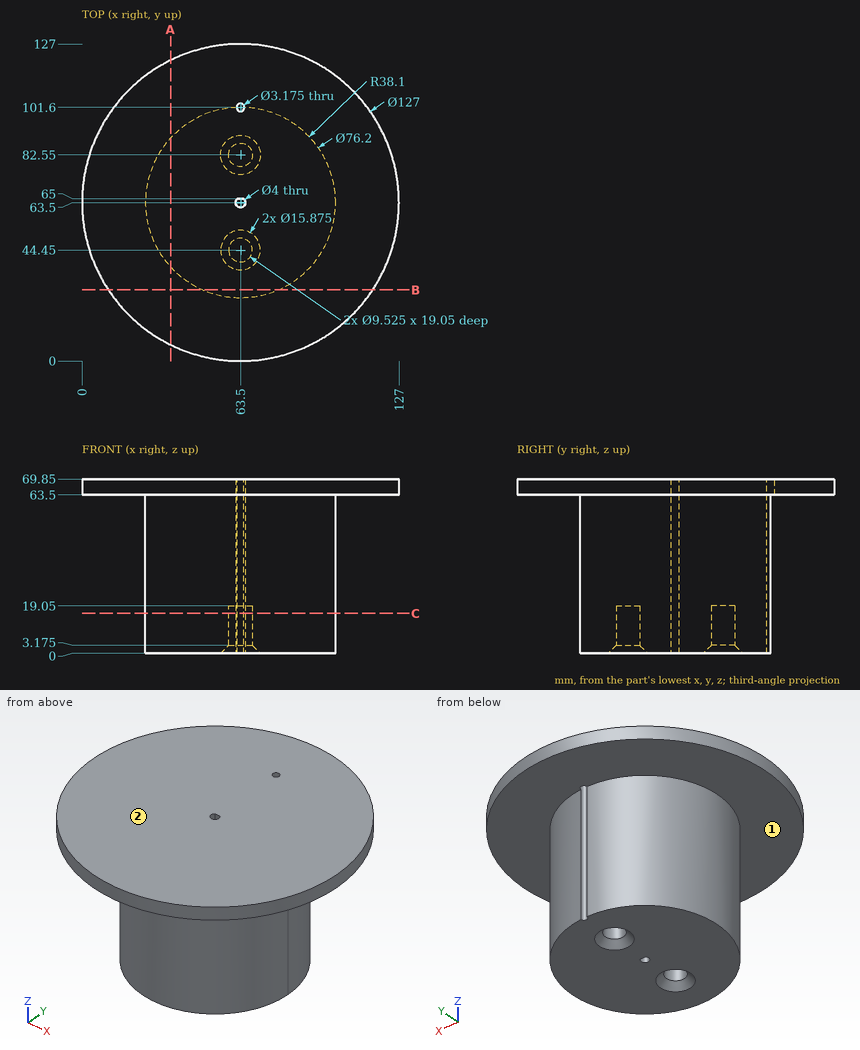
The drawing under review shows one solid part. Ordinate dimensions are in mm from its lowest x, y, z. A direction names the side the tool comes from. Coordinates: 2 decimals unless noted, no trailing zeros. Order: outer loops, then holes, each group sorted by start corner. A loop starts at its lowest first (then second) coordinate and runs counter-clockwise, first axis right, second up. Notation, with made-up numbers: (-21, -14) -> (36, -14) arc R21 ccw to (36, 13) -> close; hole circle Ø7 at (76, 51). An arc over 180 degrees is marked (long way). Answer in a Markdown table with one row per item.
(1) Wall thickness on line 1 along Y through (x, z) = (63.5, 14.25); line 2 along Y through (x, z) = (63, 11); line 3 along X through (y, z) = (63.5, 32): over which ranges is each line inside the solid? List them lowest first.
Answers:
| item | result |
|---|---|
| line 1 | 25.4 to 39.69, 49.21 to 61.5, 65 to 77.79, 87.31 to 100.01 |
| line 2 | 25.4 to 39.71, 49.19 to 61.56, 65 to 77.81, 87.29 to 100.09 |
| line 3 | 25.4 to 61.5, 65.5 to 101.6 |
(2) Insertion check: pin 1 (8 mm diameter, centred on y = 78.5, z = 33, fed in from +X); pin 2 (12 mm diameter, centred on y = 83.5, z = 17.5, fed in from -X); pin 3 (0.8 mm diameter, centred on x = 63.5, z = 31, fed in from -Y). Each pin has a flat end and moves straight along its axis. Give the tip position at first contact, or say it passes through.
Answers:
| item | result |
|---|---|
| pin 1 | x = 99.98 |
| pin 2 | x = 28.07 |
| pin 3 | y = 25.4 |
(3) Consider section A-A (x = 35.5). Write out the cut boundary in (y, z), plus the area to 3 significant figures.
Answers:
| item | result |
|---|---|
| outline | (6.51, 63.5) -> (37.66, 63.5) -> (37.66, 0) -> (89.34, 0) -> (89.34, 63.5) -> (120.49, 63.5) -> (120.49, 69.85) -> (6.51, 69.85) -> close |
| area | 4,010 mm² |
(4) Machinability: for the marked faces 1 and 2, which of the approach directions +Z, -Z, +X, -X, +Y, -Y give a long, thin tool a straight path to every point of the face, cutting with its end or side? Answer none if there is none.
Answers:
| item | result |
|---|---|
| face 1 | -Z |
| face 2 | +Z, +X, -X, +Y, -Y |
(5) Consider section C-C (z = 16). State how many separate pieces and enclosed holes the cut face has, plus the area to 3 significant figures.
Answers:
| item | result |
|---|---|
| separate pieces | 1 |
| enclosed holes | 3 |
| area | 4,400 mm² |
(6) Consider section B-B (y = 28.5). Write out the cut boundary in (x, z).
Answers:
| item | result |
|---|---|
| outline | (10.52, 63.5) -> (48.45, 63.5) -> (48.45, 0) -> (78.55, 0) -> (78.55, 63.5) -> (116.48, 63.5) -> (116.48, 69.85) -> (10.52, 69.85) -> close |
